Source: CAD feature listing. Evaluate the final solid. Frame: model axes, mm. Give positions to 0.01 mm unless a question says otherwise; leave off trailing zeros. Order: outer loops, then holes, each group sorted by start corner. A loop starts at its lowest first (then second) coordinate and runs counter-clockwise, first axis right, second up. Notation, with made-up numbers: M -27,51 L -17,51 A20 cw -17,83 Z; hole C 31.25,1.25 d6. An arc over 180 degrees is marked long. Answer in a Markdown table with one row per item. Add a question column.
(1) Pin query (flat end, axial travel): P1, Ø1.1, axis at x = 0, y = 1, coming from the +Z side; P2, Ø1.5, axis at x = -2, z = 2, coming from the -Y side; P3, Ø1.5, axis at x = -2, y = 1, coming from the +Z side; P4, Ø1.1, axis at x = 0, z = 0, coming from the -Y side. Return the tip coordinate at first contact, or that it passes through.
(2) Section query A-A, the plane y = 2.5. Return loops of the section in (x, z).
(3) Material intervals for line 1 along Z through (x, y) = (1, 1.05); line 2 along Y through (x, z) = (0.5, -1); line 3 along Z through (x, y) = (1, 2.4), sorted ascending.
(4) Mould query, pull axis X, two halves, no side actions, for faces 1 (the face through (0, 3, 0)), 2 (the face through (1.1, 1, 0)). Classes: pulls with the +X half, pulls with the -X half, needs draft (parallel to the pull), parting line crosses it, or undercut.
(5) Section query B-B, the plane y = 0.6. Return loops of the section in (x, z), plus the area to 3 significant figures.
Autodesk Inventor part; units mm, degrees
ref_plane "YZ Plane" through (0, 0, 0) normal (1, 0, 0) x (0, 1, 0)
ref_plane "XZ Plane" through (0, 0, 0) normal (0, 1, 0) x (-1, 0, 0)
ref_plane "XY Plane" through (0, 0, 0) normal (0, 0, 1) x (1, 0, 0)
sketch "Skizze1" plane through (0, 0, 0) normal (0, 1, 0) x (-1, 0, 0)
  circle A0 centre (0, 0) radius 4.039
  line L0 (0, 0) -> (1, 0)
  line L1 (1, 0) -> (1, 1)
  line L2 (1, 1) -> (0, 1)
  line L3 (0, 1) -> (0, 0)
  line L4 (1, 1) -> (-1, 1)
  line L5 (-1, 1) -> (-1, -1)
  line L6 (-1, -1) -> (1, -1)
  line L7 (1, -1) -> (1, 1)
  dimension "d10" = 1
  dimension "d11" = 1
  dimension "d12" = 2
  dimension "d13" = 2
extrude "Extrusion1" add sketch "Skizze1" along normal blind 3 contours A0 | L3 L2 L1 L0 | L0 L7 L6 L5 L4 L3
sketch "Skizze2" plane through (0, 3, 0) normal (0, 1, 0) x (1, 0, 0)
  circle A0 centre (0, 0) radius 2
extrude "Extrusion2" add sketch "Skizze2" against normal blind 1
chamfer "Fase1" distance 1.4 angle 45 1 edges at (4.039, 0, 0)
sketch "Skizze3" plane through (0, 0, 0) normal (0, -1, 0) x (1, 0, 0)
  line L0 (0, 0) -> (1.1, 0)
  line L1 (1.1, 0) -> (1.1, -1.1)
  line L2 (1.1, -1.1) -> (0, -1.1)
  line L3 (0, -1.1) -> (0, 0)
  line L4 (1.1, -1.1) -> (-1.1, -1.1)
  line L5 (-1.1, -1.1) -> (-1.1, 1.1)
  line L6 (-1.1, 1.1) -> (1.1, 1.1)
  line L7 (1.1, 1.1) -> (1.1, -1.1)
  dimension "d14" = 1.1
  dimension "d15" = 1.1
  dimension "d16" = 2.2
  dimension "d17" = 2.2
extrude "Extrusion3" cut sketch "Skizze3" against normal blind 2.7
fillet "Rundung4" radius 2 1 edges at (4.039, 3, 0)
fillet "Rundung5" radius 1 1 edges at (4.039, 1.4, 0)
properties part number "joystick" material "Gummi, Silikon"
Values follow:
| question | item | result |
|---|---|---|
| 1 | P1 | stops at z = 3.85 |
| 1 | P2 | stops at y = 0 |
| 1 | P3 | stops at z = 3.58 |
| 1 | P4 | stops at y = 2.7 |
| 2 | outline | C 0,0 d6.8; hole M -1.1,-1.1 L 1.1,-1.1 L 1.1,1.1 L -1.1,1.1 Z |
| 3 | line 1 | z = -3.53 to -1.1, 1.1 to 3.53 |
| 3 | line 2 | y = 2.7 to 3 |
| 3 | line 3 | z = -3.36 to -1.1, 1.1 to 3.36 |
| 4 | face 1 | needs draft |
| 4 | face 2 | undercut |
| 5 | outline | C 0,0 d6.48; hole M -1.1,-1.1 L 1.1,-1.1 L 1.1,1.1 L -1.1,1.1 Z |
| 5 | area | 28.1 mm² |
